```python
from build123d import *

# Parameters (mm, degrees)
BOSS_EXTRUDE1_DEPTH = 1.5
BOSS_EXTRUDE2_DEPTH = 20
LPATTERN1_COUNT     = 2
LPATTERN1_PITCH     = 40
SKETCH3_R           = 2.5
CUT_EXTRUDE1_DEPTH  = 5.238595513
CHAMFER1_SIZE       = 1


with BuildPart() as part:
    # Sketch1 → Boss-Extrude1 (new body)
    with BuildSketch(Plane(origin=(0, 0, 0), x_dir=(1, 0, 0), z_dir=(0, 1, 0))):
        with BuildLine():
            Line((-40, -17.5), (40, -17.5))
            Line((40, -17.5), (40, 12.5))
            ThreePointArc((40, 12.5), (38.535533906, 16.035533906), (35, 17.5))
            Line((35, 17.5), (-35, 17.5))
            ThreePointArc((-35, 17.5), (-38.535533906, 16.035533906), (-40, 12.5))
            Line((-40, 12.5), (-40, -17.5))
        make_face()
    extrude(amount=BOSS_EXTRUDE1_DEPTH)

    # Sketch2 → Boss-Extrude2 (add)
    with BuildSketch(Plane(origin=(40, 0, 0), x_dir=(0, 0, -1), z_dir=(1, 0, 0))):
        with BuildLine():
            Line((-17.5, 1.5), (-18.504288099, 1.5))
            ThreePointArc((-18.504288099, 1.5), (-18.842087072, 1.368635123), (-19.002386363, 1.043567414))
            ThreePointArc((-19.002386363, 1.043567414), (-23.96573551, 0.894016186), (-19.173284523, 2.193867665))
            Line((-19.173284523, 2.193867665), (-17.603081746, 2.193867665))
            ThreePointArc((-17.603081746, 2.193867665), (-25.485667036, 1.501473584), (-17.742830435, -0.13040931))
            ThreePointArc((-17.742830435, -0.13040931), (-17.669524968, -0.035807829), (-17.555328072, 0))
            Line((-17.555328072, 0), (-17.5, 0))
            Line((-17.5, 0), (-17.5, 1.5))
        make_face()
    boss_extrude2 = extrude(amount=-BOSS_EXTRUDE2_DEPTH)

    # LPattern1: Boss-Extrude2 ×2
    with Locations(*[(-i * LPATTERN1_PITCH, 0, 0) for i in range(1, LPATTERN1_COUNT)]):
        add(boss_extrude2)

    # Sketch3 → Cut-Extrude1 (cut, through all)
    with BuildSketch(Plane(origin=(0, 1.5, 0), x_dir=(1, 0, 0), z_dir=(0, 1, 0))):
        with Locations((-26, -5.5)):
            Circle(SKETCH3_R)
        with Locations((26, -5.5)):
            Circle(SKETCH3_R)
        with Locations((0, 11.85566874)):
            Circle(SKETCH3_R)
    extrude(amount=-CUT_EXTRUDE1_DEPTH, mode=Mode.SUBTRACT)

    # Chamfer1
    chamfer1_edges = [part.edges().sort_by_distance(p)[0] for p in [
        (-28.5, 1.5, 5.5),
        (23.5, 1.5, 5.5),
        (-2.5, 1.5, -11.85566874),
    ]]
    chamfer(chamfer1_edges, length=CHAMFER1_SIZE)


solid = part.part
```
The model under review builds one solid part; all positions refer to its coordinate system, in mm. A direction names the side the tool comes from. Give positions to 0.01 mm unless a question says otherwise; leave off trailing zeros. Order: outer loops, then holes, each group sorted by start corner. A loop starts at its lowest first (then second) coordinate and runs counter-clockwise, first axis right, second up. Notation, with made-up numbers: (30, 34) - (41, 34) arc R8 cw to (41, 45) - close; hole circle Ø9 at (-28, 4.25). An arc over 180 degrees is marked (long way). Use CSV: the item, a comma, the result in double quotes. Start each with the question number.
Q1. We need section A-A, the plane x = -26. Write out the cut boundary in (y, z), and give its area (3 significant figures).
Q2. We need section B-B, the plane z = 21. Write out the cut boundary in (x, y), and give its area (3 significant figures).
Q3. To check wall thickness, follow line 1 along X through (y, z) = (0.2, 5.5); line 2 along Z through (x, y) = (-26, 0.2); line 3 along Z through (x, y) = (34, 0.5). State the ranges of each line that lie inside material, in increasing order. Write a range as [from, to].
Q4. Clearance check with flat-ended pins moving along their axes: pin 1 Ø2 at (x, z) = (13, 7.5) entering from +Y; pin 2 Ø6.5 at (x, z) = (-26, 5.5) entering from +Y; pin 3 Ø0.8 at (x, y) = (-26.5, 1) entering from +Z; pin 4 Ø3 at (y, z) = (-0.5, 4.5) entering from -X. State where each tip first meets the part, or that it passes through.
Q5. We need section D-D, the plane z = -6. Write out the cut boundary in (x, y), and give its area (3 significant figures).
Q6. The part is to be moulded in two halves that separate along X. For faces 1 (the cylindrical face through (24.16, 0.25, 3.81)), 2 (the cylindrical face through (38.57, 0.74, -16)), 3 (the flat face through (0, 1, -17.5)), say which applies: +X half, -X half, draft (parallel to the pull), parting line (faces both ways), or undercut.
Q7. We need section C-C, the plane x = 26. Write out the cut boundary in (y, z), and give its area (3 significant figures).
Q8. Tool access review of faces 4 (the flat face through (30, 2.194, 18)), 5 (the flat face through (1, 0, 0)), 6 (the flat face through (0, 0, 19)), 7 (the flat face through (-20, 0, 19)): name each direction out of +Z, -Z, +X, -X, +Y, -Y from which nothing blocks a thin tool from reaching the whole face with its end or side.
Outcome:
1,outline,"(0, -17.5) - (1.5, -17.5) - (1.5, 2) - (0.5, 3) - (0, 3) - close; (0, 8) - (0.5, 8) - (1.5, 9) - (1.5, 17.5) - (0, 17.5) - close"
1,area,"44.0 mm^2"
2,outline,"(-20, -2.71) - (0, -2.71) - (0, -1.19) - (-20, -1.19) - close; (-20, 3.71) - (0, 3.71) - (0, 5.23) - (-20, 5.23) - close; (20, -2.71) - (40, -2.71) - (40, -1.19) - (20, -1.19) - close; (20, 3.71) - (40, 3.71) - (40, 5.23) - (20, 5.23) - close"
2,area,"121 mm^2"
3,line 1,"x = [-40, -28.5], [-23.5, 23.5], [28.5, 40]"
3,line 2,"z = [-17.5, 3], [8, 17.5]"
3,line 3,"z = [-17.5, 19.11], [23.87, 25.42]"
4,pin 1,"stops at y = 1.5"
4,pin 2,"stops at y = 1.25"
4,pin 3,"stops at z = 17.5"
4,pin 4,"stops at x = -40"
5,outline,"(-40, 0) - (40, 0) - (40, 1.5) - (-40, 1.5) - close"
5,area,"120 mm^2"
6,face 1,"undercut"
6,face 2,"+X half"
6,face 3,"draft"
7,outline,"(-0.13, 17.74) arc R0.2 cw to (0, 17.56) - (0, 8) - (0.5, 8) - (1.5, 9) - (1.5, 18.5) arc R0.5 ccw to (1.04, 19) arc R2.5 cw (long way) to (2.19, 19.17) - (2.19, 17.6) arc R4 ccw (long way) to start; (0, -17.5) - (1.5, -17.5) - (1.5, 2) - (0.5, 3) - (0, 3) - close"
7,area,"73.6 mm^2"
8,face 4,"-Z, +X, -X"
8,face 5,"-Z, +X, -X, -Y"
8,face 6,"+Z, +Y, -Y"
8,face 7,"+Z, -X, +Y, -Y"
